Verification items for this drawing (mm, ordinates from the low corner). Round coordinates to 2 decimals unless told otherwise and drop trailing zeros. Loops run counter-clockwise (first coordinate to the right, second up) from the corner with the lowest first, then second, coordinate; pieces in that order, holes last. Notation, with made-up numbers: M -2,80 L 8,80 A28 cw 8,114 Z; hole C -6,6 d3. An arc over 180 degrees is marked long. Answer in a Markdown table with one row per item. Add a question column.
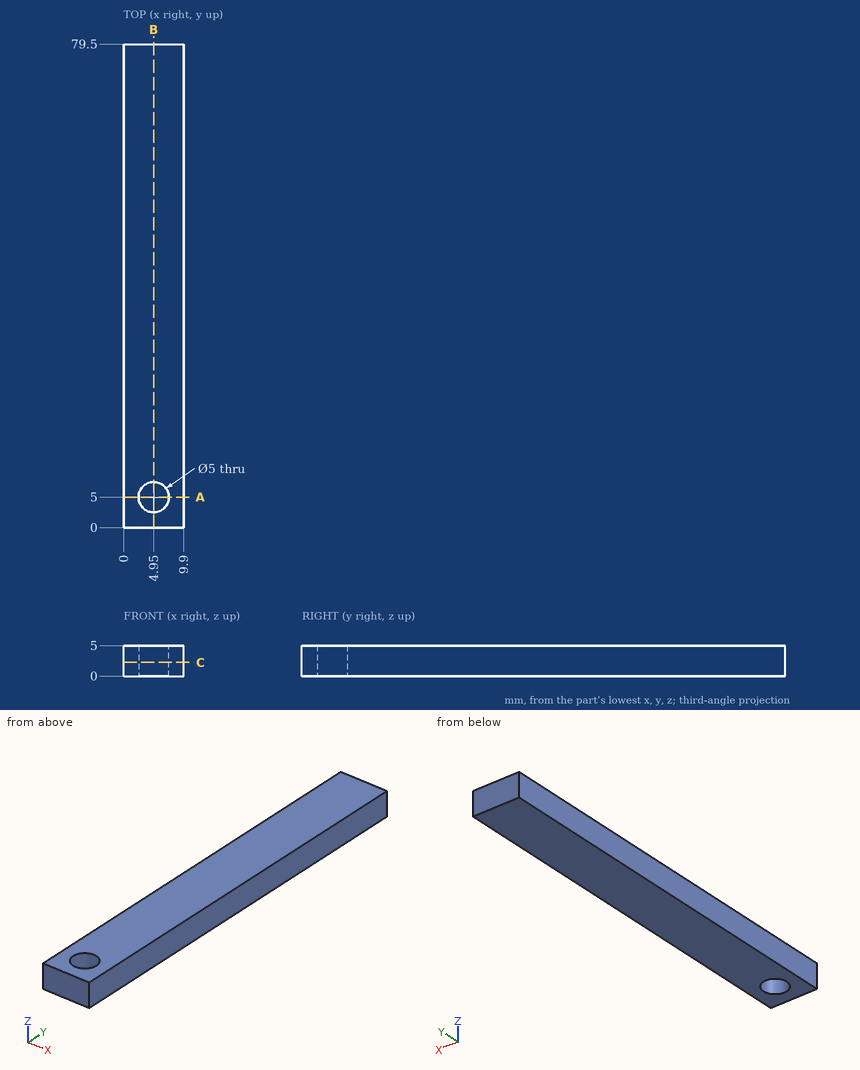
1) Cross-section at C-C, the plane z = 2.25. Record the boundary of the cut face in (x, y).
2) Thickness scan on L1, parallel to Y at x = 4.95, z = 2.2; L2, parallel to X at y = 5, z = 1.85; L3, parallel to Y at x = 3.25, z = 4.65. Record the ranges inside material, lowest first. Write a range as [from, to].
3) Cross-section at A-A, the plane y = 5. Record the boundary of the cut face in (x, z), plus the area to 3 significant figures.
4) Cross-section at B-B, the plane x = 4.95. Record the boundary of the cut face in (y, z), plus the area to 4 significant figures.
Worked answers:
| question | item | result |
|---|---|---|
| 1 | outline | M 0,0 L 9.9,0 L 9.9,79.5 L 0,79.5 Z; hole C 4.95,5 d5 |
| 2 | L1 | y = [0, 2.5], [7.5, 79.5] |
| 2 | L2 | x = [0, 2.45], [7.45, 9.9] |
| 2 | L3 | y = [0, 3.17], [6.83, 79.5] |
| 3 | outline | M 0,0 L 2.45,0 L 2.45,5 L 0,5 Z; M 7.45,0 L 9.9,0 L 9.9,5 L 7.45,5 Z |
| 3 | area | 24.5 mm2 |
| 4 | outline | M 0,0 L 2.5,0 L 2.5,5 L 0,5 Z; M 7.5,0 L 79.5,0 L 79.5,5 L 7.5,5 Z |
| 4 | area | 372.5 mm2 |
